For this review, use the dimensioned drawing (mm, ordinates from the lowest corner) and the shaded views. Give positions to 0.01 mm unless a question says otherwise; leave off trailing zeros. Order: outer loops, then holes, each group sorted by start corner. A loop starts at its lowest first (then second) coordinate and runs counter-clockwise, first axis right, second up.
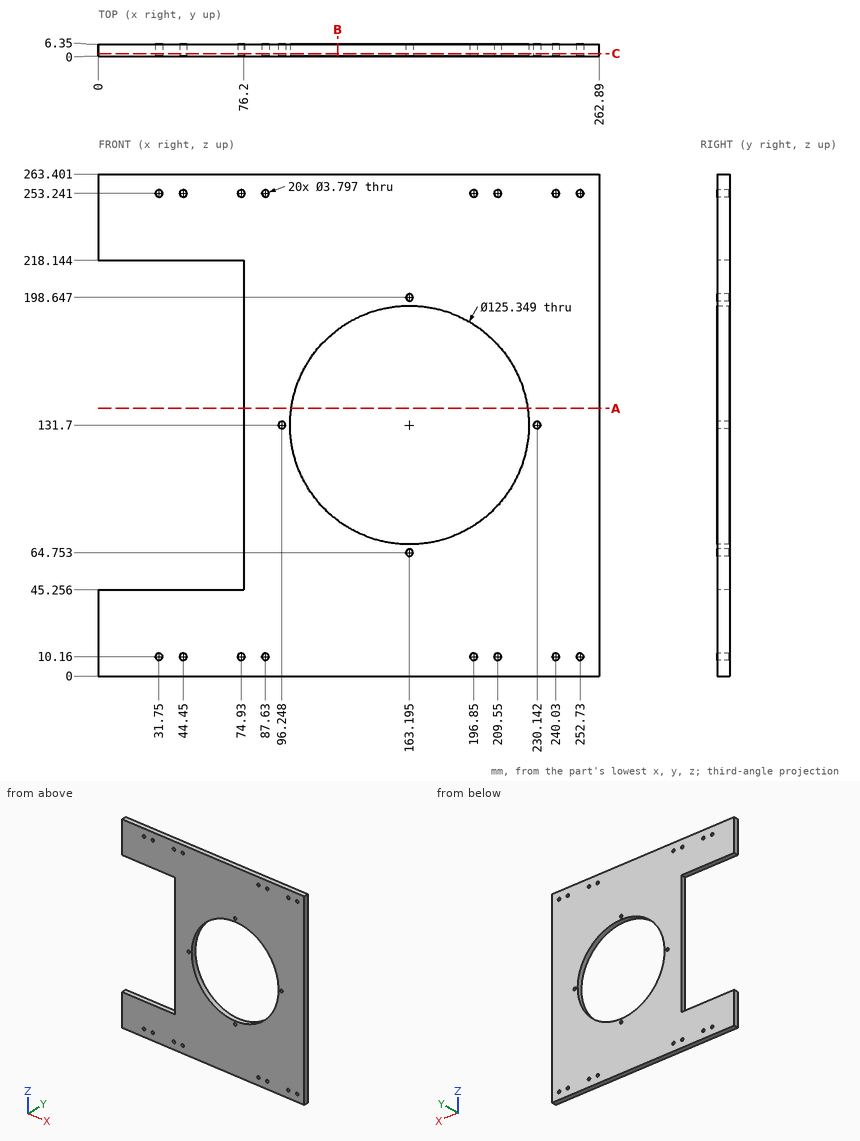
1. For pin 1 (2.5 mm diameter, centred on x = 44.45, z = 10.16, fed in from +Y); pin 2 (3 mm diameter, centred on y = 5, z = 126, fed in from -X), all flat-tipped, find the tip position at first contact; note any pin that passes through.
Recorded:
pin 1: passes through
pin 2: stops at x = 76.2
2. Take a section at B-B (x = 125.5). State the section outline as (y, z) points, then the cut area to 3 significant figures.
Recorded:
outline: (0, 0) - (6.35, 0) - (6.35, 81.63) - (0, 81.63) - close; (0, 181.77) - (6.35, 181.77) - (6.35, 263.4) - (0, 263.4) - close
area: 1,040 mm2
3. Take a section at A-A (z = 140.5). State the section outline as (x, y) points.
Recorded:
outline: (76.2, 0) - (101.14, 0) - (101.14, 6.35) - (76.2, 6.35) - close; (225.25, 0) - (262.89, 0) - (262.89, 6.35) - (225.25, 6.35) - close
4. For line 1 along Z through (x, y) = (44.45, 1.5) (1 decimal); line 2 along Z through (x, y) = (11.5, 4.75) (1 decimal); line 3 along Z through (x, y) = (196.85, 2.25), list the stretches that pass through material, from the lowest coordinate up.
Recorded:
line 1: z = 0 to 8.3, 12.1 to 45.3, 218.1 to 251.3, 255.1 to 263.4
line 2: z = 0 to 45.3, 218.1 to 263.4
line 3: z = 0 to 8.26, 12.06 to 78.83, 184.57 to 251.34, 255.14 to 263.4
5. Take a section at C-C (y = 1.25). State how many separate pieces and enclosed holes the cut face has, then the cut area to 3 significant figures.
Recorded:
separate pieces: 1
enclosed holes: 21
area: 43,500 mm2
